The model under review builds one solid part; all positions refer to its coordinate system, in mm. Coordinates: 2 decimals unless noted, no trailing zeros. Order: outer loops, then holes, each group sorted by start corner. A loop starts at its lowest first (then second) coordinate and runs counter-clockwise, first axis right, second up. Notation, with made-up numbers: M 23.5,-25.5 L 55.5,-25.5 A21 cw 55.5,0.5 Z; hole C 55.5,-14 d4. An arc over 180 degrees is marked long. Answer in a Markdown table with one row per item.
from build123d import *

# Parameters (mm, degrees)
F1_DEPTH = 28.575


with BuildPart() as f1:
    # F0 (on Top) → F1 (new body)
    with BuildSketch(Plane.XY):
        with BuildLine():
            Line((-1219.2, 457.2), (0, 457.2))
            Line((0, 457.2), (0, 609.6))
            ThreePointArc((0, 609.6), (-614.34404, 571.352323), (-1219.2, 457.2))
        make_face()
        with BuildLine():
            Line((0, 457.2), (1219.2, 457.2))
            ThreePointArc((1219.2, 457.2), (614.34404, 571.352323), (0, 609.6))
            Line((0, 609.6), (0, 457.2))
        make_face()
        Polygon((0, 0), (0, 457.2), (-1219.2, 457.2), (-1219.2, -457.2), (0, -457.2), align=None)
        Polygon((1219.2, -457.2), (1219.2, 457.2), (0, 457.2), (0, 0), (0, -457.2), align=None)
        with BuildLine():
            Line((0, -609.6), (0, -457.2))
            Line((0, -457.2), (-1219.2, -457.2))
            ThreePointArc((-1219.2, -457.2), (-614.34404, -571.352323), (0, -609.6))
        make_face()
        with BuildLine():
            ThreePointArc((0, -609.6), (614.34404, -571.352323), (1219.2, -457.2))
            Line((1219.2, -457.2), (0, -457.2))
            Line((0, -457.2), (0, -609.6))
        make_face()
    extrude(amount=F1_DEPTH)


solid = f1.part
(1) Take a section at B-B (y = 532). Write out the cut boundary in (x, z) (3 decimals), then the cut area to 3 significant figures.
Report:
| item | result |
|---|---|
| outline | M -873.318,0 L 873.318,0 L 873.318,28.575 L -873.318,28.575 Z |
| area | 49,900 mm^2 |
(2) Take a section at A-A (z = 8.75). Write out the cut boundary in (x, y).
Report:
| item | result |
|---|---|
| outline | M -1219.2,-457.2 A4953 ccw 0,-609.6 A4953 ccw 1219.2,-457.2 L 1219.2,457.2 A4953 ccw 0,609.6 A4953 ccw -1219.2,457.2 Z |
(3) Insertion check: P1, Ø1.5, axis at x = -217, y = 59.5, coming from the -Z side; P2, Ø8, axis at x = 706.5, z = 25, coming from the +Y side; P3, Ø10, axis at x = -441, z = 19, coming from the +Y side. Each pin has a flat end and moves straight along its axis. Give the tip position at first contact, or say it passes through.
Report:
| item | result |
|---|---|
| P1 | z = 0 |
| P2 | y = 559.53 |
| P3 | y = 590.37 |
(4) Take a section at C-C (x = 395.5). Write out the cut boundary in (y, z) (3 decimals).
Report:
| item | result |
|---|---|
| outline | M -593.784,0 L 593.784,0 L 593.784,28.575 L -593.784,28.575 Z |
(5) To check wall thickness, follow line 1 (Y direction, x = 560, z = 23.5); line 2 (Y direction, x = 302, z = 2.25). State the ranges of each line that lie inside material, in increasing order. Write a range as [from, to].
Report:
| item | result |
|---|---|
| line 1 | [-577.84, 577.84] |
| line 2 | [-600.38, 600.38] |
